Source: CAD feature listing. Evaluate the final solid. Frame: model axes, mm. Round coordinates to 2 decimals unless told otherwise and drop trailing zeros. Write each loop counter-clockwise with the first axis right and the second up, starting at its lowest first coordinate (ties: lowest second). Pieces come first, ordered by that corner, then holes.
from build123d import *

# Parameters (mm, degrees)
EXTRUDE_1_DEPTH = 4


with BuildPart() as part:
    # ｽｹｯﾁ1 → 押し出し-薄板1 (new body)
    with BuildSketch(Plane.XY):
        with BuildLine():
            Line((31.817918932, -48.177333301), (31.817918932, -37.177333301))
            ThreePointArc((31.817918932, -37.177333301), (13.522512959, -13.098535642), (-14.744222733, -2.35134858))
            ThreePointArc((-14.744222733, -2.35134858), (-15.865863397, -2.395137502), (-16.987504061, -2.35134858))
            ThreePointArc((-16.987504061, -2.35134858), (-18.769087239, -1.977100594), (-20.550670416, -2.35134858))
            ThreePointArc((-20.550670416, -2.35134858), (-35.568393968, -11.863545081), (-45.774892731, -26.418313577))
            ThreePointArc((-45.774892731, -26.418313577), (-46.541356838, -30.457424603), (-46.640707903, -34.567414199))
            ThreePointArc((-46.640707903, -34.567414199), (-38.091787933, -56.469515549), (-22.543394241, -74.105658262))
            ThreePointArc((-22.543394241, -74.105658262), (-19.883130575, -75.998799448), (-16.987504061, -77.507551719))
            ThreePointArc((-16.987504061, -77.507551719), (-6.850461885, -81.960889249), (3.785718261, -85.037171284))
            ThreePointArc((3.785718261, -85.037171284), (6.924298505, -85.121668583), (9.912563229, -84.158289278))
            ThreePointArc((9.912563229, -84.158289278), (23.249791669, -77.499086362), (31.664980135, -65.194158528))
            ThreePointArc((31.664980135, -65.194158528), (31.798207183, -64.69156991), (31.842654494, -64.173526282))
            Line((31.842654494, -64.173526282), (31.829698084, -53.173533912))
            Line((31.829698084, -53.173533912), (32.229697806, -53.17306277))
            Line((32.229697806, -53.17306277), (32.242654217, -64.17305514))
            ThreePointArc((32.242654217, -64.17305514), (32.192280597, -64.760171252), (32.041289943, -65.329771685))
            ThreePointArc((32.041289943, -65.329771685), (23.533127113, -77.782723155), (10.048772084, -84.538239753))
            ThreePointArc((10.048772084, -84.538239753), (6.951896278, -85.521759001), (3.703928148, -85.428738073))
            ThreePointArc((3.703928148, -85.428738073), (-6.978540006, -82.339930506), (-17.160076645, -77.868670088))
            ThreePointArc((-17.160076645, -77.868670088), (-20.096654101, -76.337084696), (-22.795002474, -74.416627193))
            ThreePointArc((-22.795002474, -74.416627193), (-38.441353007, -56.664552527), (-47.038422063, -34.618354588))
            ThreePointArc((-47.038422063, -34.618354588), (-46.939059251, -30.414609925), (-46.152726889, -26.283868638))
            ThreePointArc((-46.152726889, -26.283868638), (-35.858331906, -11.587325271), (-20.702879093, -1.981326883))
            ThreePointArc((-20.702879093, -1.981326883), (-18.799199915, -1.577194509), (-16.890627411, -1.957547479))
            ThreePointArc((-16.890627411, -1.957547479), (-15.816780094, -1.995051381), (-14.743222437, -1.950011819))
            ThreePointArc((-14.743222437, -1.950011819), (13.7790296, -12.790893821), (32.217918932, -37.10243314))
            Line((32.217918932, -37.10243314), (32.217918932, -48.177333301))
            Line((32.217918932, -48.177333301), (31.817918932, -48.177333301))
        make_face()
    extrude(amount=EXTRUDE_1_DEPTH)


solid = part.part
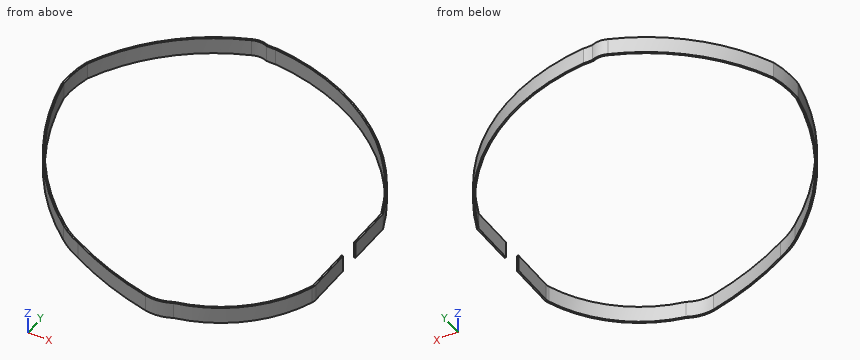
1) Section query D-D on y = -52. Return the cut outline in (x, z), then the cut area to 3 significant figures.
Taken from the geometry:
outline: (-41.04, 0) - (-40.59, 0) - (-40.59, 4) - (-41.04, 4) - close
area: 1.79 mm2
2) Contact query for flat-ended pins moving along their axis: P1, Ø1.5, axis at x = -7, z = 1, coming from the +Y side; P2, Ø2, axis at y = -75, z = 2.5, coming from the +X side; P3, Ø2, axis at y = -44, z = 2.5, coming from the +X side; P4, Ø8, axis at x = -27, y = -13, coming from the +Z side. Output: stop coordinate, or through.
Taken from the geometry:
P1: stops at y = -2.99
P2: stops at x = 27.17
P3: stops at x = 32.22
P4: passes through
3) Material intervals for line 1 (Y direction, x = 10, z = 0.35); line 2 (X direction, y = -53.5, z = 2); line 3 (Y direction, x = 27.5, z = 1.95), sorted ascending.
Taken from the geometry:
line 1: y = -84.56 to -84.14, -10.67 to -10.2
line 2: x = -40.25 to -39.8, 31.83 to 32.23
line 3: y = -73.58 to -72.92, -28.45 to -27.69
4) Section query A-A on y = -80. Return the cut outline in (x, z).
Taken from the geometry:
outline: (-12.76, 0) - (-11.77, 0) - (-11.77, 4) - (-12.76, 4) - close; (19.94, 0) - (20.66, 0) - (20.66, 4) - (19.94, 4) - close
